Build history of the part. All positions in model axes, mm. Face numbers are marked on the shaded views. A direction names the side the tool comes from. Give positions to 0.01 mm unless a question says otherwise; leave off trailing zeros. Loops run counter-clockwise (first coordinate to the right, second up) from the corner with the lowest first, then second, coordinate; pieces in that order, holes last. Notation, with made-up numbers: (-29, 1) - (-24, 1) arc R27 cw to (-24, 26) - close; hole circle Ø4 at (19.5, 38). An arc over 180 degrees is marked (long way). Return JSON: item names as keys, results as strings. Group by question number.
1) Slice it at A-A (y = 117.5). List the corners of the cut face in (x, z).
2) 3-axis set-ups, long thin cutter, end or side, ignore diameter. For the marked faces 1, 2 and 3: which of +Z, -Z, +X, -X, +Y, -Y reach the whole face in a straight line?
3) Slice it at C-C (y = 40). List the corners of the cut face in (x, z).
4) Slice it at B-B (x = -7.5). List the corners of the cut face in (y, z).
5) Drill centre lines: probe 1 along Y at (x, z) = (0, -59.35); probe 2 along X at (y, z) = (68.5, -55.25); probe 3 along Z at (x, y) = (-27, 100.5). Where is each one in solid material? Low to high. Write a range as from..to.
6) Slice it at D-D (x = 0). List the corners of the cut face in (y, z), and give its area (3 significant figures).
7) Drop flat-ended pins along their axis: pin 1 (5 mm diameter, centred on y = 74.5, z = -55, fed in from -X); pin 2 (16 mm diameter, centred on x = 15, y = 40, fed in from -Z); pin 3 (8 mm diameter, centred on x = -12, z = -51, fed in from +Y). Give the stop position or say it passes through.
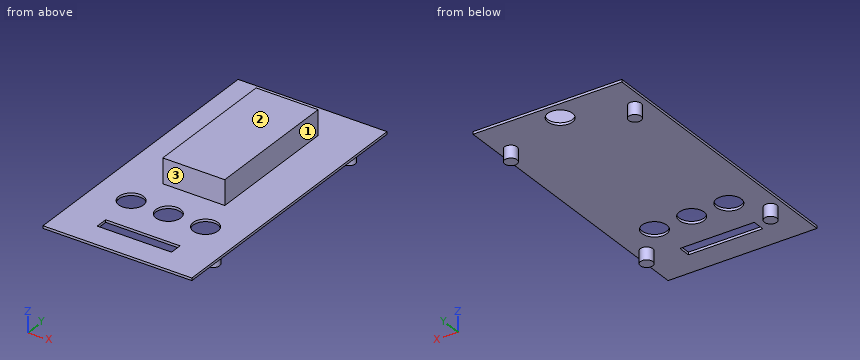
```python
from build123d import *

# Parameters (mm, degrees)
SKETCH1_R                       = 2.5
POSTS_DEPTH                     = 5
POSTS_2_DEPTH                   = 5
POSTS_3_DEPTH                   = 5
POSTS_4_DEPTH                   = 5
SKETCH2_W                       = 60
SKETCH2_H                       = 115
ELECTRONICS_CIRCUIT_BOARD_DEPTH = 1
SKETCH3_R                       = 5
SKETCH3_W                       = 30
SKETCH3_H                       = 5
MOTOR_LEADS_DEPTH               = 129.646803303
SKETCH4_W                       = 25
SKETCH4_H                       = 55
ESC_DEPTH                       = 10


with BuildPart() as part:
    # Sketch1 → Posts (new body)
    with BuildSketch(Plane.XY.offset(-65)):
        with Locations((-25, 110)):
            Circle(SKETCH1_R)
    extrude(amount=POSTS_DEPTH)



with BuildPart() as body_2:
    # Sketch1 → Posts 2 (new body)
    with BuildSketch(Plane.XY.offset(-65)):
        with Locations((25, 110)):
            Circle(SKETCH1_R)
    extrude(amount=POSTS_2_DEPTH)


with BuildPart() as body_3:
    # Sketch1 → Posts 3 (new body)
    with BuildSketch(Plane.XY.offset(-65)):
        with Locations((25, 30)):
            Circle(SKETCH1_R)
    extrude(amount=POSTS_3_DEPTH)


with BuildPart() as body_4:
    # Sketch1 → Posts 4 (new body)
    with BuildSketch(Plane.XY.offset(-65)):
        with Locations((-25, 30)):
            Circle(SKETCH1_R)
    extrude(amount=POSTS_4_DEPTH)


with BuildPart() as part_1:
    add(part.part)

    add(body_2.part)  # Electronics Circuit Board merges body 2

    add(body_3.part)  # Electronics Circuit Board merges body 3

    add(body_4.part)  # Electronics Circuit Board merges body 4
    # Sketch2 → Electronics Circuit Board (add)
    with BuildSketch(Plane.XY.offset(-60)):
        with Locations((0, 67.5)):
            Rectangle(SKETCH2_W, SKETCH2_H)
    extrude(amount=ELECTRONICS_CIRCUIT_BOARD_DEPTH)

    # Sketch3 → Motor Leads (cut, through all)
    with BuildSketch(Plane(origin=(0, 0, -60), x_dir=(-1, 0, 0), z_dir=(0, 0, -1))):
        with Locations((0, 40)):
            Circle(SKETCH3_R)
        with Locations((-15, 40)):
            Circle(SKETCH3_R)
        with Locations((15, 40)):
            Circle(SKETCH3_R)
        with Locations((0, 117.5)):
            Circle(SKETCH3_R)
        with Locations((0, 22.5)):
            Rectangle(SKETCH3_W, SKETCH3_H)
    extrude(amount=-MOTOR_LEADS_DEPTH, mode=Mode.SUBTRACT)

    # Sketch4 → ESC (add)
    with BuildSketch(Plane.XY.offset(-59)):
        with Locations((0, 82.5)):
            Rectangle(SKETCH4_W, SKETCH4_H)
    extrude(amount=ESC_DEPTH)


solid = part_1.part
```
Results:
{
 "1": {"outline": "(-30, -60) - (-5, -60) - (-5, -59) - (-30, -59) - close; (5, -60) - (30, -60) - (30, -59) - (5, -59) - close"},
 "2": {"face 1": "+Z, +X, +Y, -Y", "face 2": "+Z, +X, -X, +Y, -Y", "face 3": "+Z, +X, -X, -Y"},
 "3": {"outline": "(-30, -60) - (-20, -60) - (-20, -59) - (-30, -59) - close; (-10, -60) - (-5, -60) - (-5, -59) - (-10, -59) - close; (5, -60) - (10, -60) - (10, -59) - (5, -59) - close; (20, -60) - (30, -60) - (30, -59) - (20, -59) - close"},
 "4": {"outline": "(10, -60) - (20, -60) - (20, -59) - (10, -59) - close; (25, -60) - (125, -60) - (125, -59) - (110, -59) - (110, -49) - (55, -49) - (55, -59) - (25, -59) - close"},
 "5": {"probe 1": "10..20, 25..35, 45..112.5, 122.5..125", "probe 2": "-12.5..12.5", "probe 3": "-60..-59"},
 "6": {"outline": "(10, -60) - (20, -60) - (20, -59) - (10, -59) - close; (25, -60) - (35, -60) - (35, -59) - (25, -59) - close; (45, -60) - (112.5, -60) - (112.5, -59) - (110, -59) - (110, -49) - (55, -49) - (55, -59) - (45, -59) - close; (122.5, -60) - (125, -60) - (125, -59) - (122.5, -59) - close", "area": "640 mm2"},
 "7": {"pin 1": "x = -12.5", "pin 2": "z = -60", "pin 3": "y = 110"}
}
